The model under review builds one solid part; all positions refer to its coordinate system, in mm. Face numbers are marked on the shaded views. A direction names the side the tool comes from. Round coordinates to 2 decimals unless told otherwise and drop trailing zeros. Loops run counter-clockwise (first coordinate to the right, second up) from the corner with the lowest first, then second, coordinate; pieces in that order, holes last. Notation, with made-up numbers: (8, 21) -> (44, 21) arc R6 ccw to (44, 28) -> close; hole circle Ø8 at (55, -25.75). An arc over 180 degrees is marked (long way). Write each question's results on one line, items separated by ' | '. Start each with the question number.
Item 1: Clearance check with flat-ended pins moving along their axes: pin 1 Ø12 at (x, z) = (0.5, 15.5) entering from -Y; pin 2 Ø1.5 at (y, z) = (48.5, 7) entering from -X; pin 3 Ø4 at (x, z) = (-2, -4.5) entering from -Y; pin 4 Ø0.5 at (x, y) = (4, 8.5) entering from -Z. State where each tip first meets the part, or that it passes through.
Item 2: We need section D-D (y = 6.5). Give the boundary of the cut face in (x, z), and give its area (3 significant figures).
Item 3: We need section A-A (y = 20). Give the boundary of the cut face in (x, z), and give its area (3 significant figures).
Item 4: We need section B-B (z = -16.75). Give the number of separate pieces and of enclosed holes in the cut face, and give its area (3 significant figures).
Item 5: Mouldability with a two-part tool opening along X and no side actions: class the marked faces 4, 5 and 6 as pulls with the +X half, pulls with the -X half, needs draft (parallel to the pull), parting line crosses it, or undercut.
Item 6: Tool access review of the marked faces 1, 2 and 3: name each direction out of +Z, -Z, +X, -X, +Y, -Y from which nothing blocks a thin tool from reaching the whole face with its end or side.
Item 7: For L1, parallel to Y at x = 14.5, z = 16.75; L2, parallel to X at y = 11, z = 4; L3, parallel to Y at x = 14, z = 16, list the stretches that pass through material, from the lowest coordinate up. Write a range as from..to.
from build123d import *

# Parameters (mm, degrees)
RESSALTO_EXTRUS_O1_DEPTH   = 55
ESBO_O2_W                  = 26
ESBO_O2_H                  = 17.5
CORTE_EXTRUS_O1_DEPTH      = 52
CORTE_EXTRUS_O2_DEPTH      = 29.5
ESBO_O4_W                  = 23
ESBO_O4_H                  = 10
CORTE_EXTRUS_O3_DEPTH      = 52
ESBO_O5_W                  = 20
ESBO_O5_H                  = 16
CORTE_EXTRUS_O4_DEPTH      = 52
RESSALTO_EXTRUS_O3_DEPTH   = 9
RESSALTO_EXTRUS_O4_DEPTH   = 9
CORTE_EXTRUS_O7_DEPTH      = 62.227546905
ESBO_O12_R                 = 1.6
CORTE_EXTRUS_O8_DEPTH      = 66.930360988
CORTE_EXTRUS_O9_DEPTH      = 67.479320093
CORTE_EXTRUS_O9_DEPTH_BACK = 67.479320093


with BuildPart() as part:
    # Esboço1 → Ressalto-extrusão1 (new body)
    with BuildSketch(Plane(origin=(0, 0, 0), x_dir=(1, 0, 0), z_dir=(0, 1, 0))):
        with BuildLine():
            Line((15, 12.25), (16.5, 12.25))
            Line((16.5, 12.25), (16.5, 10.75))
            Line((16.5, 10.75), (16.5, -10.75))
            Line((16.5, -10.75), (16.5, -12.25))
            Line((16.5, -12.25), (15, -12.25))
            Line((15, -12.25), (-15, -12.25))
            ThreePointArc((-15, -12.25), (-16.060660172, -11.810660172), (-16.5, -10.75))
            Line((-16.5, -10.75), (-16.5, 10.75))
            ThreePointArc((-16.5, 10.75), (-16.060660172, 11.810660172), (-15, 12.25))
            Line((-15, 12.25), (15, 12.25))
        make_face()
    extrude(amount=RESSALTO_EXTRUS_O1_DEPTH)

    # Esboço2 → Corte-extrusão1 (cut)
    with BuildSketch(Plane(origin=(0, 55, 0), x_dir=(1, 0, 0), z_dir=(0, 1, 0))):
        Rectangle(ESBO_O2_W, ESBO_O2_H)
    extrude(amount=-CORTE_EXTRUS_O1_DEPTH, mode=Mode.SUBTRACT)

    # Esboço3 → Corte-extrusão2 (cut)
    with BuildSketch(Plane.ZY.offset(16.5)):
        Polygon((-4.25, 8), (0.75, 8), (0.75, 3), (-4.25, 3), (-12.25, 3), (-12.25, 8), align=None)
    extrude(amount=-CORTE_EXTRUS_O2_DEPTH, mode=Mode.SUBTRACT)

    # Esboço4 → Corte-extrusão3 (cut)
    with BuildSketch(Plane(origin=(0, 0, -12.25), x_dir=(-1, 0, 0), z_dir=(0, 0, -1))):
        with Locations((0, 17.5)):
            Rectangle(ESBO_O4_W, ESBO_O4_H)
        with Locations((0, 31.5)):
            Rectangle(ESBO_O4_W, ESBO_O4_H)
        with BuildLine():
            Line((11.5, 40.5), (24.942410125, 40.5))
            Line((24.942410125, 40.5), (24.942410125, 59.834456184))
            Line((24.942410125, 59.834456184), (-1.5, 59.834456184))
            Line((-1.5, 59.834456184), (-6.076098787, 62.09241335))
            Line((-6.076098787, 62.09241335), (-7.576098787, 62.09241335))
            Line((-7.576098787, 62.09241335), (-7.576098787, 57.63082944))
            Line((-7.576098787, 57.63082944), (-16.5, 57.63082944))
            Line((-16.5, 57.63082944), (-16.5, 55))
            Line((-16.5, 55), (-7.576098787, 55))
            Line((-7.576098787, 55), (-7.157696235, 55))
            ThreePointArc((-7.157696235, 55), (-6.380774636, 54.702427517), (-5.834045456, 54.07533601))
            ThreePointArc((-5.834045456, 54.07533601), (0.640063345, 44.48758485), (11.5, 40.5))
        make_face()
    extrude(amount=-CORTE_EXTRUS_O3_DEPTH, mode=Mode.SUBTRACT)

    # Esboço5 → Corte-extrusão4 (cut)
    with BuildSketch(Plane.XZ):
        Rectangle(ESBO_O5_W, ESBO_O5_H)
    extrude(amount=-CORTE_EXTRUS_O4_DEPTH, mode=Mode.SUBTRACT)

    # Esboço6 → Ressalto-extrusão3 (add)
    with BuildSketch(Plane(origin=(0, 0, -12.25), x_dir=(-1, 0, 0), z_dir=(0, 0, -1))):
        Polygon((-16.5, 55), (-13, 55), (-13, 40), (-8.260417548, 40), (15, 40), (15, 37), (-8.260417548, 37), (-13, 37), (-13, 26), (-8.260417548, 26), (15, 26), (15, 23), (-8.260417548, 23), (-13, 23), (-13, 12), (-8.260417548, 12), (15, 12), (15, 9), (-8.260417548, 9), (-13, 9), (-13, 3), (15, 3), (15, 0), (-16.5, 0), align=None)
    extrude(amount=RESSALTO_EXTRUS_O3_DEPTH)

    # Esboço9 → Ressalto-extrusão4 (add)
    with BuildSketch(Plane.XY.offset(12.25)):
        Polygon((13, 23), (13, 12), (8.260417548, 12), (-15, 12), (-15, 9), (8.260417548, 9), (13, 9), (13, 3), (-15, 3), (-15, 0), (16.5, 0), (16.5, 55), (13, 55), (13, 40), (8.260417548, 40), (-15, 40), (-15, 37), (8.260417548, 37), (13, 37), (13, 26), (8.260417548, 26), (-15, 26), (-15, 23), (8.260417548, 23), align=None)
    extrude(amount=RESSALTO_EXTRUS_O4_DEPTH)

    # Esboço11 → Corte-extrusão7 (cut, through all)
    with BuildSketch(Plane(origin=(0, 55, 0), x_dir=(1, 0, 0), z_dir=(0, 1, 0))):
        Polygon((13, 21.25), (-15, 12.25), (-18.396269007, 13.557013), (-20.171014906, 2.968836485), (-21.687729599, -13.92980577), (-19.283641957, -16.807997198), (-15, -12.25), (13, -21.25), (12.387270144, -22.842176527), (-13.733579981, -25.767037441), (-25.593893111, -17.703590231), (-24.101496534, -8.799916531), (-21.404407074, 21.25), (-11.342896145, 26.819075861), (13.346838628, 26.819075861), align=None)
    extrude(amount=-CORTE_EXTRUS_O7_DEPTH, mode=Mode.SUBTRACT)

    # Esboço12 → Corte-extrusão8 (cut, through all)
    with BuildSketch(Plane.ZY.offset(-13)):
        with Locations((-16.75, 45)):
            Circle(ESBO_O12_R)
        with Locations((-16.75, 31.5)):
            Circle(ESBO_O12_R)
        with Locations((-16.75, 17.5)):
            Circle(ESBO_O12_R)
        with Locations((16.75, 17.5)):
            Circle(ESBO_O12_R)
        with Locations((16.75, 31.5)):
            Circle(ESBO_O12_R)
        with Locations((16.75, 45)):
            Circle(ESBO_O12_R)
    extrude(amount=-CORTE_EXTRUS_O8_DEPTH, mode=Mode.SUBTRACT)

    # Esboço13 → Corte-extrusão9 (cut, two sides: drawn at the far end of the back side and taken through both)
    with BuildSketch(Plane(origin=(0, 0, -12.25), x_dir=(-1, 0, 0), z_dir=(0, 0, -1)).offset(-CORTE_EXTRUS_O9_DEPTH_BACK)):
        Polygon((-16, 57.748375369), (-15.75, 57.748375369), (-15.75, -2.748375369), (-16, -2.748375369), (-16.5, -2.748375369), (-21.567741729, -3.81911432), (-26.240802846, 1.764024497), (-29.75124657, 11.630119118), (-32.031223005, 26.530526522), (-32.963463423, 30.826938884), (-36.481605691, 47.040985858), align=None)
        Polygon((16.5, -3.81911432), (16, -3.81911432), (15.75, -9.987267399), (15.75, 53.083012796), (16, 53.083012796), (35.334385386, 35.109894688), (36.940493813, 23.637691641), (28.756988973, 6.505868423), align=None)
    extrude(amount=CORTE_EXTRUS_O9_DEPTH + CORTE_EXTRUS_O9_DEPTH_BACK, mode=Mode.SUBTRACT)


solid = part.part
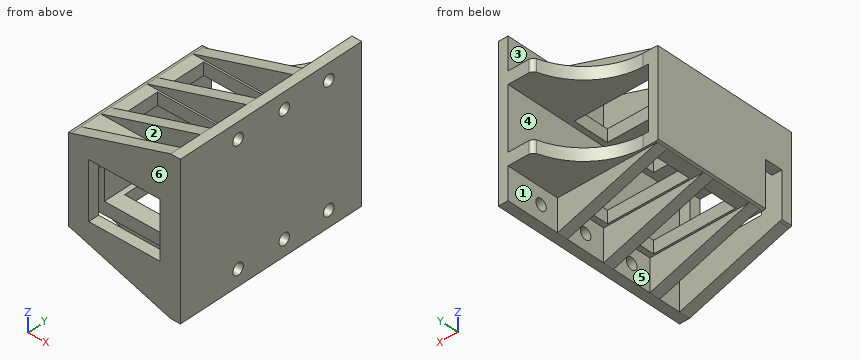
Here are the results:
1) pin 1: stops at y = 0 | pin 2: stops at x = 13 | pin 3: passes through | pin 4: stops at z = -12.25
2) outline: (-15.75, 0.75) -> (-13, 0.75) -> (-13, 8.75) -> (13, 8.75) -> (13, -21.25) -> (15.75, -21.25) -> (15.75, 21.25) -> (13, 21.25) -> (13, 12.25) -> (-15, 12.25) arc R1.5 ccw to (-15.75, 12.05) -> close | area: 239 mm2
3) outline: (-15.75, -12.05) arc R1.5 ccw to (-15, -12.25) -> (-11.5, -12.25) -> (-11.5, -8.75) -> (-13, -8.75) -> (-13, 8.75) -> (-11.5, 8.75) -> (-11.5, 12.25) -> (-15, 12.25) arc R1.5 ccw to (-15.75, 12.05) -> close; (11.5, -12.25) -> (13, -12.25) -> (13, -21.25) -> (15.75, -21.25) -> (15.75, 21.25) -> (13, 21.25) -> (13, 12.25) -> (11.5, 12.25) -> (11.5, 8.75) -> (13, 8.75) -> (13, -8.75) -> (11.5, -8.75) -> close | area: 205 mm2
4) separate pieces: 4 | enclosed holes: 0 | area: 293 mm2
5) face 4: undercut | face 5: pulls with the -X half | face 6: needs draft
6) face 1: -Z, -X, +Y | face 2: +Z, -X | face 3: +Z, -X, +Y
7) L1: y = 0..15.9, 19.1..29.9, 33.1..43.4, 46.6..55 | L2: x = -15.75..-13, 13..15.75 | L3: y = 0..16.09, 18.91..30.09, 32.91..43.59, 46.41..55
